from build123d import *

# Parameters (mm, degrees)
EXTRUDE_1_DEPTH     = 38
SKETCH_2_W          = 70
SKETCH_2_H          = 28
CUT_EXTRUDE_1_DEPTH = 21
SKETCH_3_R          = 1.65
SKETCH_3_W          = 42
SKETCH_3_H          = 21
CUT_EXTRUDE_2_DEPTH = 20
SKETCH_5_R          = 1.65
CUT_EXTRUDE_3_DEPTH = 10
SKETCH_7_W          = 55
SKETCH_7_H          = 25.515470347
CUT_EXTRUDE_4_DEPTH = 2.5
FILLET_1_R          = 3
FILLET_2_R          = 0.5
SKETCH_8_R          = 1.35
SKETCH_8_W          = 22
SKETCH_8_H          = 4
CUT_EXTRUDE_5_DEPTH = 5


with BuildPart() as part:
    # 草图1 → 凸台-拉伸1 (new body)
    with BuildSketch(Plane.XY):
        Polygon((7, 0), (63, 0), (70, 7), (70, 18), (63, 25), (7, 25), (0, 18), (0, 7), align=None)
    extrude(amount=EXTRUDE_1_DEPTH)

    # 草图2 → 切除-拉伸1 (cut)
    with BuildSketch(Plane(origin=(0, 25, 0), x_dir=(1, 0, 0), z_dir=(0, 1, 0))):
        with Locations((35, -19)):
            Rectangle(SKETCH_2_W, SKETCH_2_H)
    extrude(amount=-CUT_EXTRUDE_1_DEPTH, mode=Mode.SUBTRACT)

    # 草图3 → 切除-拉伸2 (cut)
    with BuildSketch(Plane.XY.offset(38)):
        with Locations((12.5, 19.5)):
            Circle(SKETCH_3_R)
        with Locations((12.5, 9.5)):
            Circle(SKETCH_3_R)
        with Locations((61.5, 19.5)):
            Circle(SKETCH_3_R)
        with Locations((61.5, 9.5)):
            Circle(SKETCH_3_R)
        with Locations((36.5, 14.5)):
            Rectangle(SKETCH_3_W, SKETCH_3_H)
    extrude(amount=-CUT_EXTRUDE_2_DEPTH, mode=Mode.SUBTRACT)

    # 草图5 → 切除-拉伸3 (cut)
    with BuildSketch(Plane(origin=(0, 0, 0), x_dir=(-1, 0, 0), z_dir=(0, 0, -1))):
        with Locations((-22.5, 14.5)):
            Circle(SKETCH_5_R)
        with Locations((-47.5, 14.5)):
            Circle(SKETCH_5_R)
    extrude(amount=-CUT_EXTRUDE_3_DEPTH, mode=Mode.SUBTRACT)

    # 草图7 → 切除-拉伸4 (cut)
    with BuildSketch(Plane.XY.offset(38)):
        with Locations((37, 16.757735174)):
            Rectangle(SKETCH_7_W, SKETCH_7_H)
    extrude(amount=-CUT_EXTRUDE_4_DEPTH, mode=Mode.SUBTRACT)

    # 圆角1
    fillet_1_edges = [part.edges().sort_by_distance(p)[0] for p in [
        (63, 25, 34.25),
        (0, 7, 35.5),
        (0, 18, 35.5),
        (7, 25, 35.5),
        (70, 18, 35.5),
        (70, 7, 35.5),
        (63, 0, 19),
        (7, 0, 19),
        (0, 7, 2.5),
        (0, 18, 2.5),
        (63, 25, 2.5),
        (70, 18, 2.5),
        (70, 7, 2.5),
    ]]
    fillet(fillet_1_edges, radius=FILLET_1_R)

    # 圆角2
    fillet_2_edges = [part.edges().sort_by_distance(p)[0] for p in [
        (8.871320344, 25, 38),
        (66.810660172, 21.189339828, 38),
        (34.378679656, 25, 0),
        (3.5, 3.5, 0),
        (0, 12.5, 0),
        (66.5, 21.5, 0),
        (70, 12.5, 0),
        (66.5, 3.5, 0),
        (35, 0, 0),
        (7.09459039, 0.228361402, 0),
        (0.228361402, 7.09459039, 0),
        (0.228361402, 17.90540961, 0),
        (62.90540961, 0.228361402, 0),
        (69.771638598, 7.09459039, 0),
        (69.771638598, 17.90540961, 0),
        (62.90540961, 24.771638598, 0),
        (70, 12.5, 38),
        (3.5, 21.5, 38),
        (0, 12.5, 38),
        (3.5, 3.5, 38),
        (35, 0, 38),
        (66.5, 3.5, 38),
        (7.09459039, 0.228361402, 38),
        (0.228361402, 7.09459039, 38),
        (0.228361402, 17.90540961, 38),
        (7.09459039, 24.771638598, 38),
        (62.90540961, 0.228361402, 38),
        (69.771638598, 7.09459039, 38),
        (69.771638598, 17.90540961, 38),
        (3.939339828, 21.939339828, 0),
    ]]
    fillet(fillet_2_edges, radius=FILLET_2_R)

    # 草图8 → 切除-拉伸5 (cut, through all)
    with BuildSketch(Plane(origin=(0, 4, 0), x_dir=(1, 0, 0), z_dir=(0, 1, 0))):
        with Locations((35, -11.5)):
            Circle(SKETCH_8_R)
        with Locations((35, -33.5)):
            Circle(SKETCH_8_R)
        with Locations((35, -7)):
            Rectangle(SKETCH_8_W, SKETCH_8_H)
    extrude(amount=-CUT_EXTRUDE_5_DEPTH, mode=Mode.SUBTRACT)


solid = part.part
Verification items for the finished model (mm, model axes). A direction names the side the tool comes from. Round coordinates to 2 decimals unless told otherwise and drop trailing zeros. Loops run counter-clockwise (first coordinate to the right, second up) from the corner with the lowest first, then second, coordinate; pieces in that order, holes last. Notation, with made-up numbers: (-4.5, 0.5) - (7.5, 0.5) arc R16 cw to (7.5, 19.5) - close; hole circle Ø3 at (-9.75, -40). An arc over 180 degrees is marked (long way). Use a Markdown table: item, result. Add a question column.
1. Section check A-A, the plane x = 12.5. Record the boundary of the cut face in (y, z).
2. Section check C-C, the plane x = 22.5. Record the boundary of the cut face in (y, z).
3. Access from +Z, -Z, +X, -X, +Y, -Y to the whole of each face (thin tool, end or side, straight path). Record for faces 1 (the face through (64.5, 14, 37)), 2 (the face through (46, 2, 7)), 3 (the face through (59.85, 19.57, 34.27)).
4. Gauge pin test, flat ends, axial feed: pin 1 (3 mm diameter, centred on x = 61.5, y = 19.5, fed in from +Z); pin 2 (6 mm diameter, centred on x = 24.5, y = 7.5, fed in from -Z); pin 3 (4.5 mm diameter, centred on x = 61.5, y = 9.5, fed in from +Z); pin 4 (2 mm diameter, centred on x = 19, z = 34, fed in from +Y). Record the tip position at first contact, or that the pin passes through.
5. Section check B-B, the plane z = 11.5. Record the boundary of the cut face in (x, y).
6. Release check for a two-part mould opening along Y. For faces 4 (the face through (49.15, 14.57, 2.46)), 5 (the face through (13.39, 20.89, 34.27)), 6 (the face through (61, 15, 35.5)), 7 (the face through (4, 22, 35)) record: released by +Y, released by -Y, zero draft, split by the parting line, or undercut.
7. Thickness scan on probe 1 along Z at (x, y) = (35, 0.9); probe 2 along Y at (x, z) = (12.5, 34.9); probe 3 along Z at (x, y) = (7.5, 23.75). Record the ranges inside material, lowest first. Write a range as [from, to].
8. Section check D-D, the plane y = 14.5. Record the boundary of the cut face in (x, z), plus the area to 3 significant figures.
Checks:
| question | item | result |
|---|---|---|
| 1 | outline | (0, 0.5) arc R0.5 ccw to (0.5, 0) - (24.5, 0) arc R0.5 ccw to (25, 0.5) - (25, 5) - (4, 5) - (4, 33) - (7.85, 33) - (7.85, 35.5) - (4, 35.5) - (4, 38) - (0.5, 38) arc R0.5 ccw to (0, 37.5) - close; (11.15, 33) - (17.85, 33) - (17.85, 35.5) - (11.15, 35.5) - close; (21.15, 33) - (25, 33) - (25, 35.5) - (21.15, 35.5) - close |
| 2 | outline | (0, 0.5) arc R0.5 ccw to (0.5, 0) - (12.85, 0) - (12.85, 5) - (4, 5) - (4, 38) - (0.5, 38) arc R0.5 ccw to (0, 37.5) - close; (16.15, 0) - (24.5, 0) arc R0.5 ccw to (25, 0.5) - (25, 5) - (16.15, 5) - close |
| 3 | face 1 | +Z, +Y |
| 3 | face 2 | +Y, -Y |
| 3 | face 3 | +Z |
| 4 | pin 1 | stops at z = 5 |
| 4 | pin 2 | stops at z = 0 |
| 4 | pin 3 | stops at z = 35.5 |
| 4 | pin 4 | stops at y = 4 |
| 5 | outline | (3, 4) - (6.12, 0.88) arc R3 ccw to (8.24, 0) - (33.65, 0) - (33.65, 4) - close; (36.35, 0) - (61.76, 0) arc R3 ccw to (63.88, 0.88) - (67, 4) - (36.35, 4) - close |
| 6 | face 4 | undercut |
| 6 | face 5 | undercut |
| 6 | face 6 | zero draft |
| 6 | face 7 | released by +Y |
| 7 | probe 1 | z = [0, 5], [9, 10.15], [12.85, 32.15], [34.85, 38] |
| 7 | probe 2 | y = [0, 7.85], [11.15, 17.85], [21.15, 25] |
| 7 | probe 3 | z = [0, 5], [33, 38] |
| 8 | outline | (0, 0.5) arc R0.5 ccw to (0.5, 0) - (20.85, 0) - (20.85, 5) - (0, 5) - close; (0, 33) - (15.5, 33) - (15.5, 35.5) - (9.5, 35.5) - (9.5, 38) - (0.5, 38) arc R0.5 ccw to (0, 37.5) - close; (24.15, 0) - (45.85, 0) - (45.85, 5) - (24.15, 5) - close; (49.15, 0) - (69.5, 0) arc R0.5 ccw to (70, 0.5) - (70, 5) - (49.15, 5) - close; (57.5, 33) - (70, 33) - (70, 37.5) arc R0.5 ccw to (69.5, 38) - (64.5, 38) - (64.5, 35.5) - (57.5, 35.5) - close |
| 8 | area | 424 mm^2 |
